Could you check a few things on this drawing? It's one solid part, dimensions in mm from its lowest x, y, z. A direction names the side the tool comes from. Coordinates: 2 decimals unless noted, no trailing zeros. Write each loop counter-clockwise with the first axis right and the second up, starting at its lowest first coordinate (ties: lowest second). Pieces come first, ordered by that corner, then holes. Notation, with made-up numbers: (-11.5, -33) - (19.5, -33) arc R24 ccw to (19.5, -3) - close; hole circle Ø4 at (-35.75, 6). An arc over 180 degrees is marked (long way). Use one line per item in the form item = value. Start each with the question number.
(1) On a 3-axis mill with a long thin cutter (end or side, diameter ignored), from which of +Z, -Z, +X, -X, +Y, -Y can I reach the whole of each face in a straight line? I mean the marked faces 1 and 2. Say none if no direction works.
(2) If I drill on probe 1 along Z at (x, y) = (2.75, 2.65) (1 decimal); probe 2 along X at (y, z) = (2.2, 9); probe 3 along Z at (x, y) = (12.25, 2.1) (1 decimal), over which ranges is the centre line in solid material (lowest first)? Write a range as from..to.
(3) If we section it at A-A on y = 2: Give the number of separate pieces and of enclosed holes in the cut face.
(4) If we section it at D-D on z = 11.5: Please give me the cut outline in (x, y), then the cut area to 3 significant figures.
(5) If we section it at B-B on x = 4: Please give me the cut outline in (y, z) (1 decimal).
(6) For pin 1 Ø3 at (x, z) = (3, 3) entering from -Y; pin 2 Ø1 at (y, z) = (2.5, 6) entering from +X; pin 3 Ø0.9 at (y, z) = (1.5, 13.5) entering from +X; pin 4 Ø3 at (x, z) = (15.5, 17.5) entering from -Y, each with a flat end and sliding along its axis, tell me the tip position at first contact or that it passes through.
(7) Thinking about a two-plate mould opening in X: for the marked faces 3, 4, 5 and 6, which applies, pulls with the +X half, pulls with the -X half, needs draft (parallel to the pull), parting line crosses it, or undercut?
(8) If we section it at C-C on z = 20.75: Please give me the cut outline in (x, y) (1 decimal).
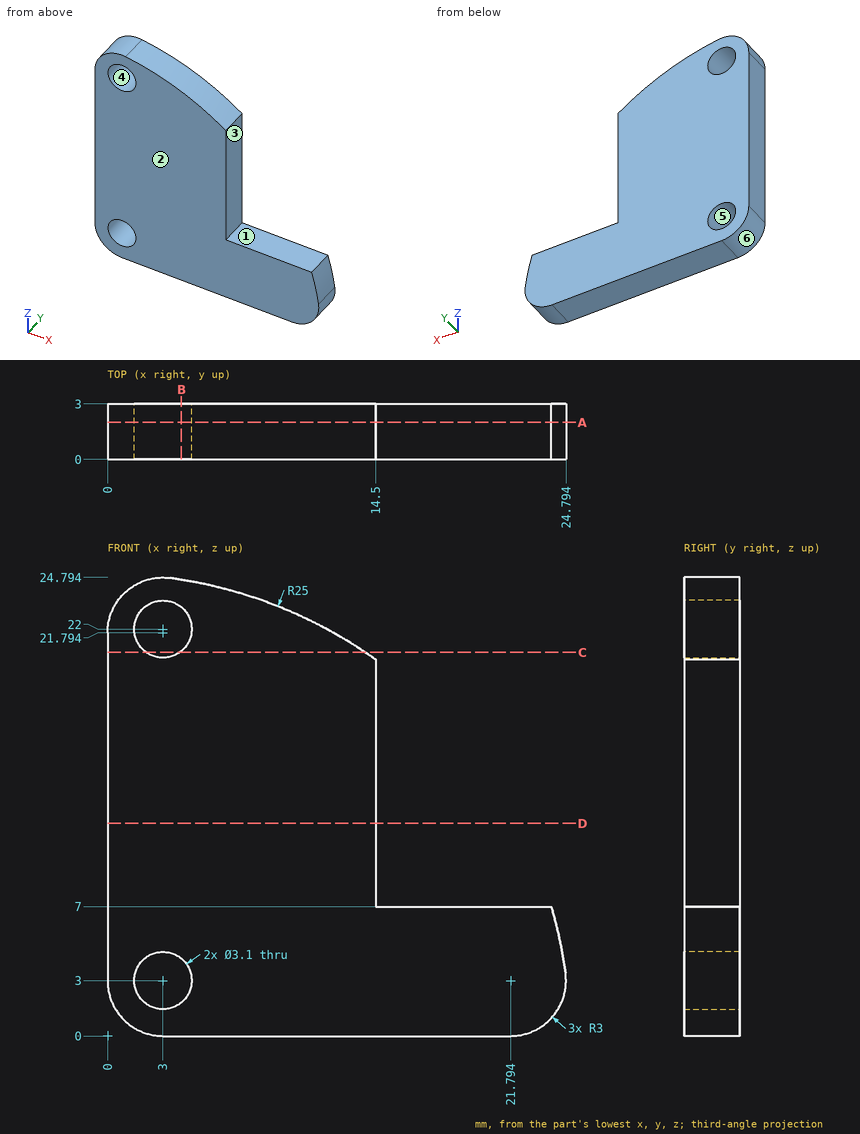
Reported:
q1.face_1 = +Z, +X, +Y, -Y
q1.face_2 = +Z, -Z, +X, -X, -Y
q2.probe_1 = 0..1.5, 4.5..20.5, 23.5..24.8
q2.probe_2 = 0..14.5
q2.probe_3 = 0..21.8
q3.separate_pieces = 1
q3.enclosed_holes = 2
q4.outline = (0, 0) - (14.5, 0) - (14.5, 3) - (0, 3) - close
q4.area = 43.5 mm2
q5.outline = (0, 0) - (3, 0) - (3, 1.8) - (0, 1.8) - close; (0, 4.2) - (3, 4.2) - (3, 20.8) - (0, 20.8) - close; (0, 23.2) - (3, 23.2) - (3, 24.7) - (0, 24.7) - close
q6.pin_1 = through
q6.pin_2 = 24.39
q6.pin_3 = 14.5
q6.pin_4 = 0
q7.face_3 = pulls with the +X half
q7.face_4 = undercut
q7.face_5 = undercut
q7.face_6 = pulls with the -X half
q8.outline = (0, 0) - (2.1, 0) - (2.1, 3) - (0, 3) - close; (3.9, 0) - (13.9, 0) - (13.9, 3) - (3.9, 3) - close
